Here's the drawing with two shaded views (mm, measured from the low corner). I have some questions. A direction names the side the tool comes from. Coordinates: 2 decimals unless noted, no trailing zeros. Write each loop counter-clockwise with the first axis right and the second up, starting at its lowest first coordinate (ties: lowest second). Pieces come first, ordered by that corner, then holes. Notation, with made-up numbers: (56.25, -12) -> (76.25, -12) arc R25 cw to (76.25, 16) -> close; hole circle Ø5 at (28, 13). An arc over 180 degrees is marked (long way). Answer in a Markdown table with one row per item. Add a question column.
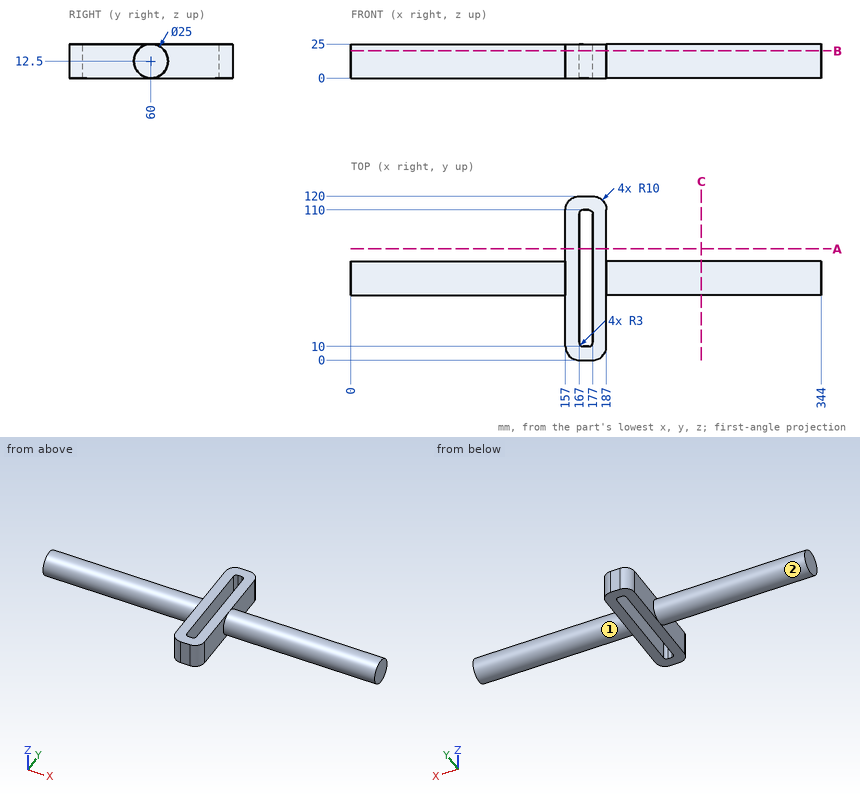
Q1. Imagine slicing it at B-B on z = 20. Please give me the cut outline in (x, y).
Q2. I'm going to push flat-ended pins straight in: P1, Ø8, axis at x = 210, y = 77.5, coming from the -Z side; P2, Ø1, axis at y = 89, z = 3.5, coming from the -X side; P3, Ø8, axis at x = 201, y = 55, coming from the +Z side; P4, Ø2, axis at x = 216, z = 4, coming from the +Y side. Where does each tip first touch, or does it pass through?
Q3. Imagine slicing it at C-C on x = 256.5. Please give me the cut outline in (y, z), plus the area to 3 significant figures.
Q4. I need wall thicknesses on line 1 (X direction, y = 91.5, z = 7); line 2 (X direction, y = 55.5, z = 7.5); line 3 (Y direction, x = 222, z = 12.75). Which ranges of each line are inside material? Lowest first, please. Write a range as [from, to].
Q5. Imagine slicing it at A-A on y = 81.5. Please give me the cut outline in (x, z), plus the area to 3 significant figures.
Q6. For the marked faces 1 and 2, which set-ups out of +Z, -Z, +X, -X, +Y, -Y let a thin tool reach every point of the face, with its end or its side?
Result sheet:
| question | item | result |
|---|---|---|
| 1 | outline | (0, 50) -> (157, 50) -> (157, 10) arc R10 ccw to (167, 0) -> (177, 0) arc R10 ccw to (187, 10) -> (187, 50) -> (344, 50) -> (344, 70) -> (187, 70) -> (187, 110) arc R10 ccw to (177, 120) -> (167, 120) arc R10 ccw to (157, 110) -> (157, 70) -> (0, 70) -> close; hole (167, 13) arc R3 ccw to (170, 10) -> (174, 10) arc R3 ccw to (177, 13) -> (177, 107) arc R3 ccw to (174, 110) -> (170, 110) arc R3 ccw to (167, 107) -> close |
| 2 | P1 | passes through |
| 2 | P2 | stops at x = 157 |
| 2 | P3 | stops at z = 24.96 |
| 2 | P4 | stops at y = 70 |
| 3 | outline | circle Ø25 at (60, 12.5) |
| 3 | area | 491 mm^2 |
| 4 | line 1 | x = [157, 167], [177, 187] |
| 4 | line 2 | x = [0, 167], [177, 344] |
| 4 | line 3 | y = [47.5, 72.5] |
| 5 | outline | (157, 0) -> (167, 0) -> (167, 25) -> (157, 25) -> close; (177, 0) -> (187, 0) -> (187, 25) -> (177, 25) -> close |
| 5 | area | 500 mm^2 |
| 6 | face 1 | +X |
| 6 | face 2 | -X |
